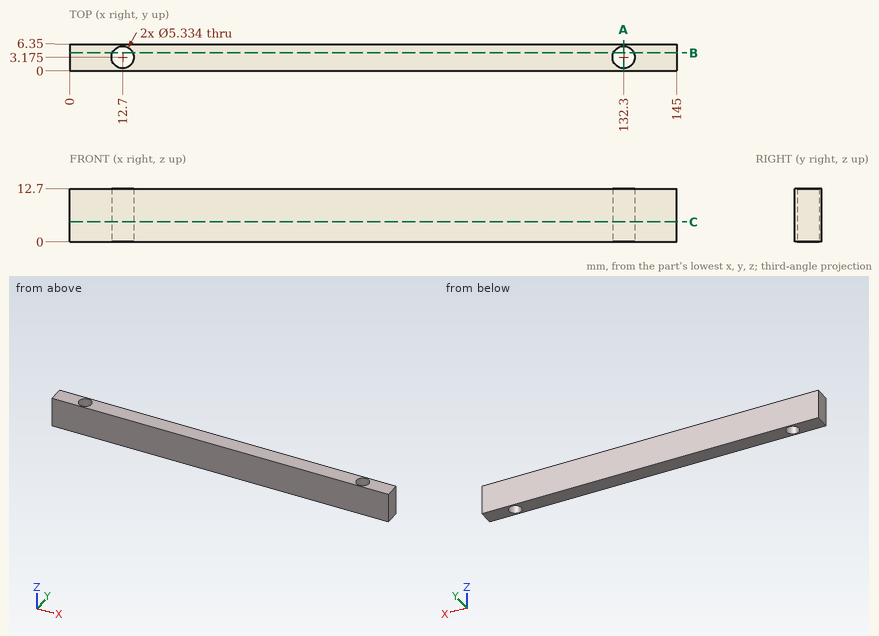
Input: dimensioned drawing with shaded views. Units: mm. Origin: part minimum x, y, z. Give positions to 0.01 mm unless a question says otherwise; leave off trailing zeros. Loops run counter-clockwise (first coordinate to the right, second up) from the corner with the lowest first, then second, coordinate; pieces in that order, holes last. Notation, with made-up numbers: M -25,0 L -21,0 A20 cw -21,24 Z; hole C 16.5,-13 d7. An arc over 180 degrees is marked long. Put each result on its own line as item: value. Start each with the question number.
1) Cut plane A-A (x = 132.3). Output: boundary loops of the cut face in (y, z), then the cut area to 3 significant figures.
2) Cut plane C-C (z = 4.75). Output: boundary loops of the cut face in (x, y) (3 decimals).
3) Contact query for a flat-ended pin moving along its axis: pin 1 (6 mm diameter, centred on x = 113.5, z = 6, fed in from -Y). Output: stop coordinate, or through.
4) Ray query, line 1 along Y through (x, z) = (132.3, 9); line 2 along X through (y, z) = (4, 11.5); line 3 along X through (y, z) = (2, 5.25). Return the intervals inside material, ascending.
5) Cut plane B-B (y = 4.25). Output: boundary loops of the cut face in (x, z).
Verdict:
1. outline: M 0,0 L 0.51,0 L 0.51,12.7 L 0,12.7 Z; M 5.84,0 L 6.35,0 L 6.35,12.7 L 5.84,12.7 Z
1. area: 12.9 mm2
2. outline: M 0,0 L 145,0 L 145,6.35 L 0,6.35 Z; hole C 12.7,3.175 d5.334; hole C 132.3,3.175 d5.334
3. pin 1: y = 0
4. line 1: 0 to 0.51, 5.84 to 6.35
4. line 2: 0 to 10.16, 15.24 to 129.76, 134.84 to 145
4. line 3: 0 to 10.31, 15.09 to 129.91, 134.69 to 145
5. outline: M 0,0 L 10.26,0 L 10.26,12.7 L 0,12.7 Z; M 15.14,0 L 129.86,0 L 129.86,12.7 L 15.14,12.7 Z; M 134.74,0 L 145,0 L 145,12.7 L 134.74,12.7 Z
